Check sheet for the modelled part. Datum: model origin and axes. Units: mm. A direction names the side the tool comes from. Round coordinates to 2 decimals unless told otherwise and drop trailing zeros. Write each loop counter-clockwise with the first axis right and the second up, starting at its lowest first coordinate (ties: lowest second). Pieces come first, ordered by that corner, then holes. Notation, with made-up numbers: (-33, 11.25) -> (22, 11.25) arc R18 ccw to (22, 41.25) -> close; hole circle Ø4 at (-36, 8.5). An arc over 180 degrees is marked (long way). One line per item, written item: value.
from build123d import *

# Parameters (mm, degrees)
RIB9_REACH        = 80.502
SKETCH5_WALL_W    = 189.003354934
SKETCH5_WALL_H    = 6
CIRPATTERN1_COUNT = 4


with BuildPart() as part:
    # Sketch1 → Revolve2 (revolve)
    with BuildSketch(Plane.XY, mode=Mode.PRIVATE) as revolve2_sk:
        with BuildLine():
            ThreePointArc((-56.342741935, -0.846438172), (-48.342741935, 7.153561828), (-56.342741935, 15.153561828))
            Line((-56.342741935, 15.153561828), (-56.342741935, 21.153561828))
            ThreePointArc((-56.342741935, 21.153561828), (-42.342741935, 7.153561828), (-56.342741935, -6.846438172))
            Line((-56.342741935, -6.846438172), (-56.342741935, -0.846438172))
        make_face()
        with BuildLine():
            Line((-17.342741935, -14.846438172), (-17.342741935, 26.153561828))
            Line((-17.342741935, 26.153561828), (-26.342741935, 26.153561828))
            Line((-26.342741935, 26.153561828), (-26.342741935, 21.153561828))
            Line((-26.342741935, 21.153561828), (-26.342741935, 18.153561828))
            Line((-26.342741935, 18.153561828), (-26.342741935, 10.153561828))
            Line((-26.342741935, 10.153561828), (-42.667947604, 10.153561828))
            ThreePointArc((-42.667947604, 10.153561828), (-42.342741935, 7.153561828), (-42.667947604, 4.153561828))
            Line((-42.667947604, 4.153561828), (-26.342741935, 4.153561828))
            Line((-26.342741935, 4.153561828), (-26.342741935, -3.846438172))
            Line((-26.342741935, -3.846438172), (-26.342741935, -6.846438172))
            Line((-26.342741935, -6.846438172), (-26.342741935, -14.846438172))
            Line((-26.342741935, -14.846438172), (-17.342741935, -14.846438172))
        make_face()
    revolve(revolve2_sk.sketch.rotate(Axis((-8.342741935, 57.152217742, 0), (0, -1, 0)), 270), axis=Axis((-8.342741935, 57.152217742, 0), (0, -1, 0)))

    # Sketch5 wall → Rib9 (add, up to next)
    with BuildSketch(Plane(origin=(-41.342741935, 21.153561828, 0), x_dir=(-1, 0, 0), z_dir=(0, -1, 0)), mode=Mode.PRIVATE) as rib9_sk1:
        Rectangle(SKETCH5_WALL_W, SKETCH5_WALL_H)
    rib9_tool1 = extrude(rib9_sk1.sketch, amount=RIB9_REACH, mode=Mode.PRIVATE) - part.part
    rib9 = rib9_tool1.solids().sort_by_distance((-41.342741935, 21.153561828, 0))[0]
    add(rib9)

    # CirPattern1: Rib9 ×4 about axis
    cirpattern1_axis = Axis((-8.342741935, 0, 0), (0, 1, 0))
    for i in range(1, CIRPATTERN1_COUNT):
        add(rib9.rotate(cirpattern1_axis, i * 360 / CIRPATTERN1_COUNT))

    # Mirror1: part across plane


with BuildPart() as part_1:
    add(part.part)
    add(part.part.mirror(Plane.ZX.offset(7.153561828)))


solid = part_1.part
Item 1: Sectioned sample at B-B on y = 17. Enter the section's corners in (x, z), and give its area (3 significant figures).
Answer:
outline: circle Ø96 at (-8.34, 0); hole (-46.27, -3) arc R38.05 ccw to (-11.34, -37.93) -> (-11.34, -17.75) arc R18 cw to (-26.09, -3) -> close; hole (-46.27, 3) -> (-26.09, 3) arc R18 cw to (-11.34, 17.75) -> (-11.34, 37.93) arc R38.05 ccw to start; hole circle Ø18 at (-8.34, 0); hole (-5.34, -37.93) arc R38.05 ccw to (29.59, -3) -> (9.41, -3) arc R18 cw to (-5.34, -17.75) -> close; hole (-5.34, 17.75) arc R18 cw to (9.41, 3) -> (29.59, 3) arc R38.05 ccw to (-5.34, 37.93) -> close
area: 3,940 mm^2
Item 2: Mould release check, pull along Z, two halves, no side actions. Record for faces 5 (the flat face through (-11.343, 16, 29)), 6 (the flat face through (-17, 29.154, 4)): pulls with the +Z half, pulls with the -Z half, needs draft (parallel to the pull), parting line crosses it, or undercut.
Answer:
face 5: undercut
face 6: needs draft
Item 3: Sectioned sample at D-D on y = 24. Enter the section's corners in (x, z).
Answer:
outline: circle Ø36 at (-8.34, 0); hole circle Ø18 at (-8.34, 0)
Item 4: Sectioned sample at C-C on y = -5. Enter the section's corners in (x, z), and give its area (3 significant figures).
Answer:
outline: circle Ø96 at (-8.34, 0); hole (-49.28, -3) arc R41.05 ccw to (-11.34, -40.94) -> (-11.34, -17.75) arc R18 cw to (-26.09, -3) -> close; hole (-49.28, 3) -> (-26.09, 3) arc R18 cw to (-11.34, 17.75) -> (-11.34, 40.94) arc R41.05 ccw to start; hole circle Ø18 at (-8.34, 0); hole (-5.34, -40.94) arc R41.05 ccw to (32.6, -3) -> (9.41, -3) arc R18 cw to (-5.34, -17.75) -> close; hole (-5.34, 17.75) arc R18 cw to (9.41, 3) -> (32.6, 3) arc R41.05 ccw to (-5.34, 40.94) -> close
area: 3,260 mm^2
Item 5: Depth check by flat-ended pin: P1, Ø5, axis at x = -7.5, z = -36, coming from the +Y side; P2, Ø12, axis at y = -1, z = 30, coming from the -X side; P3, Ø6, axis at x = -20, y = 22, coming from the -Z side. Enter the tip coordinate at first touch or a pass-through.
Answer:
P1: stops at y = 21.15
P2: stops at x = -49.91
P3: stops at z = -47.19
Item 6: Sectioned sample at A-A on z = 0. Enter the section's corners in (x, y), and give its area (3 significant figures).
Answer:
outline: (-56.34, -6.85) -> (-26.34, -6.85) -> (-26.34, -14.85) -> (-17.34, -14.85) -> (-17.34, 29.15) -> (-26.34, 29.15) -> (-26.34, 21.15) -> (-56.34, 21.15) -> (-56.34, 15.15) arc R8 cw to (-56.34, -0.85) -> close; (0.66, -14.85) -> (9.66, -14.85) -> (9.66, -6.85) -> (39.66, -6.85) -> (39.66, -0.85) arc R8 cw to (39.66, 15.15) -> (39.66, 21.15) -> (9.66, 21.15) -> (9.66, 29.15) -> (0.66, 29.15) -> close
area: 2,270 mm^2
Item 7: Thickness scan on line 1 (X direction, y = -4, z = 19); line 2 (X direction, y = -10.5, z = 0.5); line 3 (X direction, y = 16, z = -23). Record the ranges inside material, lowest first.
Answer:
line 1: x = -52.42 to -43.02, -11.34 to -5.34, 26.33 to 35.74
line 2: x = -26.34 to -17.33, 0.64 to 9.65
line 3: x = -50.47 to -37.52, -11.34 to -5.34, 20.83 to 33.79
Item 8: Tool access check on faces 1 (the flat face through (-27, 4.154, -18)), 2 (the flat face through (-8, 21.154, -33)), 3 (the flat face through (24, 21.154, 0)), 4 (the flat face through (-11.343, 16, -29)). Record the directions out of +Z, -Z, +X, -X, +Y, -Y that give a thin tool (end or side, any length) a straight path to the whole face; none if there is none.
Answer:
face 1: -Y
face 2: -Z, +X, -X, +Y
face 3: +Z, -Z, +X, +Y
face 4: +Y
